```python
from build123d import *

# Parameters (mm, degrees)
F0_W     = 30
F0_H     = 30
F1_DEPTH = 30
F2_R     = 14.99999
F3_W     = 4.3548396789
F3_H     = 1.9354838878
F4_DEPTH = 40
F5_R     = 2


# Not quite as in the source:
# - a fillet or chamfer is up to 0.001 mm smaller than in the source, because OpenCascade refuses the exact size
# - the program builds the solid bodies; features that only make, move or delete a surface that nothing else refers to are left out


with BuildPart() as f1:
    # F0 (on Top) → F1 (new body)
    with BuildSketch(Plane.XY):
        Rectangle(F0_W, F0_H)
    extrude(amount=F1_DEPTH)

    # F2 (radius 15 in the source; OpenCascade refuses exactly that, so slightly less here)
    f2_edges = [f1.edges().sort_by_distance(p)[0] for p in [
        (-15, -15, 15),
        (-15, 0, 30),
        (0, -15, 30),
        (0, 15, 30),
        (15, 0, 30),
        (15, 15, 15),
        (-15, 15, 15),
        (0, 15, 0),
        (-15, 0, 0),
        (0, -15, 0),
        (15, 0, 0),
        (15, -15, 15),
    ]]
    fillet(f2_edges, radius=F2_R)

    # F3 (on Top) → F4 (join)
    with BuildSketch(Plane.XY):
        with Locations((3.7499994505, 4.5967744663)):
            Rectangle(F3_W, F3_H)
        with Locations((-5.3500005495, 4.5967744663)):
            Rectangle(F3_W, F3_H)
    extrude(amount=F4_DEPTH)

    # F5
    f5_edges = [f1.edges().sort_by_distance(p)[0] for p in [
        (5.927419, 4.596774, 40),
        (-3.172581, 4.596774, 40),
        (1.57258, 4.596774, 40),
        (-7.52742, 4.596774, 40),
    ]]
    fillet(f5_edges, radius=F5_R)


solid = f1.part
```
The listing builds one solid part. Answer for the finished solid, in the listing's coordinates (mm). A direction names the side the tool comes from. Give positions to 0.01 mm unless a question says otherwise; leave off trailing zeros. Loops run counter-clockwise (first coordinate to the right, second up) from the corner with the lowest first, then second, coordinate; pieces in that order, holes last. Notation, with made-up numbers: (42, 54.25) - (99, 54.25) arc R25 cw to (99, 79.25) - close; hole circle Ø8 at (57.5, -12.5). An arc over 180 degrees is marked (long way). Return JSON: item names as keys, results as strings. Group by question number.
1. Given pin 1 Ø2 at (x, z) = (-6, 32.5) entering from -Y; pin 2 Ø12 at (y, z) = (-1.5, 7) entering from +X; pin 3 Ø2 at (y, z) = (4, 1) entering from +X; pin 4 Ø8 at (x, y) = (0.5, 7.5) entering from +Z, each flat-ended and moving along its own axis, determine where each tip first touches the part or whether it passes through.
2. Which of the six approach directions +Z, -Z, +X, -X, +Y, -Y give full straight-line access (tool end or side, diameter ignored) to faces 1 (the flat face through (-7.527, 5, 1)), 2 (the cylindrical face through (2.143, 4.61, 39.399)), 3 (the cylindrical face through (5.357, 4.61, 39.399))?
3. Straight lines are drawn through the part: line 1 (Z direction, x = 5, y = -4); line 2 (X direction, y = 13.5, z = 15); line 3 (Y direction, x = 4, z = 29.5). For each, find the intervals that lie inside material, in ascending order. Write a range as [from, to].
4. Determine the mould class of faces 4 (the flat face through (-6, 3.629, 1)), 5 (the cylindrical face through (-3.743, 4.61, 39.399)), 6 (the flat face through (-5, 5.565, 33)) for opening direction Y: pulls with the +Y half, pulls with the -Y half, needs draft (parallel to the pull), parting line crosses it, or undercut.
5. Find section A-A (z = 34.5). Write down the section's boundary in (x, y), then the cut area to 3 significant figures.
Verdict:
{
 "1": {"pin 1": "stops at y = 3.63", "pin 2": "stops at x = 14.85", "pin 3": "stops at x = 6.41", "pin 4": "stops at z = 40"},
 "2": {"face 1": "-Z, -X, +Y", "face 2": "+Z, +Y, -Y", "face 3": "+Z, +X, +Y, -Y"},
 "3": {"line 1": "z = [1.44, 28.56]", "line 2": "x = [-6.54, 6.54]", "line 3": "y = [3.63, 5.56]"},
 "4": {"face 4": "undercut", "face 5": "needs draft", "face 6": "pulls with the +Y half"},
 "5": {"outline": "(-7.53, 3.63) - (-3.17, 3.63) - (-3.17, 5.56) - (-7.53, 5.56) - close; (1.57, 3.63) - (5.93, 3.63) - (5.93, 5.56) - (1.57, 5.56) - close", "area": "16.9 mm^2"}
}
